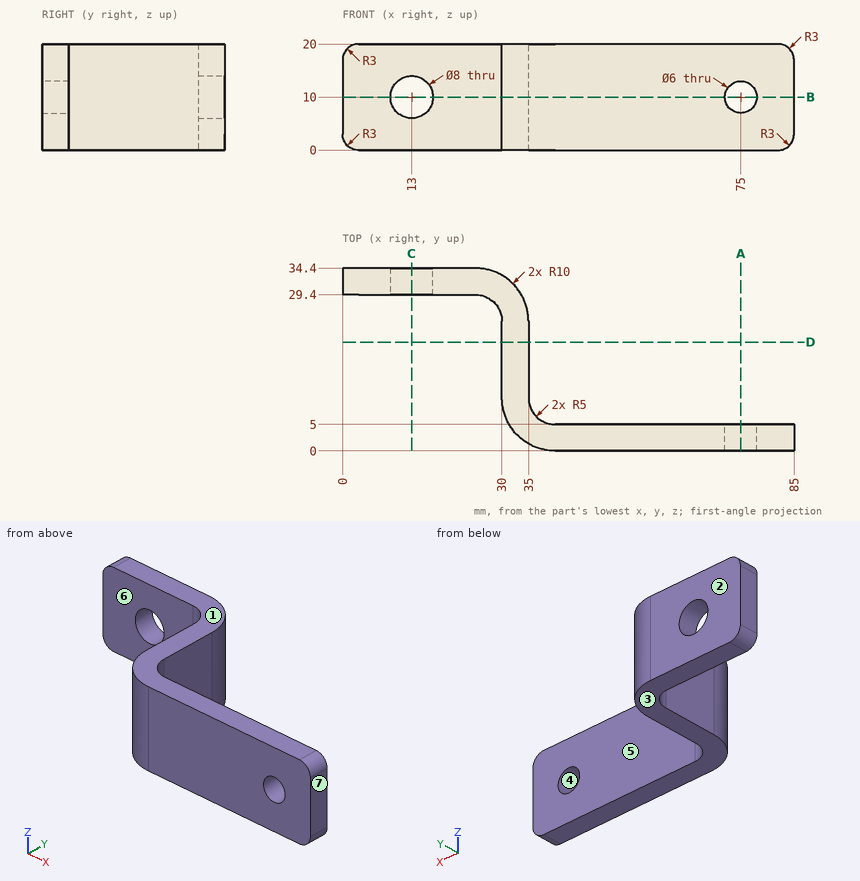
Verification items for this drawing (mm, ordinates from the low corner). A direction names the side the tool comes from. Coordinates: 2 decimals unless noted, no trailing zeros. Loops run counter-clockwise (first coordinate to the right, second up) from the corner with the lowest first, then second, coordinate; pieces in that order, holes last. Notation, with made-up numbers: (56, 9.5) - (62, 9.5) arc R21 cw to (62, 34.5) - close; hole circle Ø8 at (39, 87.25). An arc over 180 degrees is marked (long way). Use one line per item in the form item = value. Start each with the question number.
Item 1: Section check D-D, the plane y = 20.5. Enter the section's corners in (x, z).
Item 2: Tool access check on the marked faces 5, 6 and 7. Record the directions out of +Z, -Z, +X, -X, +Y, -Y that give a thin tool (end or side, any length) a straight path to the whole face; none if there is none.
Item 3: Section check B-B, the plane z = 10. Enter the section's corners in (x, y), and give its area (3 significant figures).
Item 4: Gauge pin test, flat ends, axial feed: pin 1 (4 mm diameter, centred on x = 58, z = 14.5, fed in from +Y); pin 2 (1 mm diameter, centred on y = 26.5, z = 18, fed in from -X); pin 3 (8 mm diameter, centred on y = 18, z = 6, fed in from +X). Record the tip position at first contact, or that the pin passes through.
Item 5: Mould release check, pull along Z, two halves, no side actions. Record for the marked faces 1, 2, 3 and 4: +Z half, -Z half, draft (parallel to the pull), parting line (faces both ways), or undercut.
Item 6: Thickness scan on probe 1 along X at (y, z) = (21, 14); probe 2 along Y at (x, z) = (5, 9.75); probe 3 along Y at (x, z) = (55, 10.25). Record the ranges inside material, lowest first.
Item 7: Section check A-A, the plane x = 75. Enter the section's corners in (y, z).
Item 8: Section check C-C, the plane x = 13. Enter the section's corners in (y, z), and give its area (3 significant figures).
Computed:
q1.outline = (30, 0) - (35, 0) - (35, 20) - (30, 20) - close
q2.face_5 = +Z, -Z, +X, +Y
q2.face_6 = +Z, -Z, -X, -Y
q2.face_7 = +Z, -Z, +X, +Y, -Y
q3.outline = (0, 29.4) - (9, 29.4) - (9, 34.4) - (0, 34.4) - close; (17, 29.4) - (25, 29.4) arc R5 cw to (30, 24.4) - (30, 10) arc R10 ccw to (40, 0) - (72, 0) - (72, 5) - (40, 5) arc R5 cw to (35, 10) - (35, 24.4) arc R10 ccw to (25, 34.4) - (17, 34.4) - close; (78, 0) - (85, 0) - (85, 5) - (78, 5) - close
q3.area = 470 mm2
q4.pin_1 = 5
q4.pin_2 = 29.27
q4.pin_3 = 35
q5.face_1 = +Z half
q5.face_2 = draft
q5.face_3 = -Z half
q5.face_4 = undercut
q6.probe_1 = 30 to 35
q6.probe_2 = 29.4 to 34.4
q6.probe_3 = 0 to 5
q7.outline = (0, 0) - (5, 0) - (5, 7) - (0, 7) - close; (0, 13) - (5, 13) - (5, 20) - (0, 20) - close
q8.outline = (29.4, 0) - (34.4, 0) - (34.4, 6) - (29.4, 6) - close; (29.4, 14) - (34.4, 14) - (34.4, 20) - (29.4, 20) - close
q8.area = 60.0 mm2
